```python
from build123d import *

# Parameters (mm, degrees)
EXTRUDE_1_DEPTH        = 2.9
SKETCH_2_R             = 2.75
EXTRUDE_2_DEPTH        = 5
FILLET_2_R             = 0.7
HOLE_WIZARD_M3_1_D     = 2.5
HOLE_WIZARD_M3_1_DEPTH = 10.1
HOLE_WIZARD_M3_1_TIP   = 0.751075774
FILLET_4_R             = 0.2


with BuildPart() as part:
    # 草图1 → 凸台-拉伸1 (new body)
    with BuildSketch(Plane(origin=(0, 0, 0), x_dir=(1, 0, 0), z_dir=(0, 1, 0))):
        Polygon((2.75, -1.58771324), (2.75, 1.58771324), (0, 3.175426481), (-2.75, 1.58771324), (-2.75, -1.58771324), (0, -3.175426481), align=None)
    extrude(amount=EXTRUDE_1_DEPTH)

    # 草图2 → 凸台-拉伸2 (add)
    with BuildSketch(Plane(origin=(0, 0, 0), x_dir=(-1, 0, 0), z_dir=(0, -1, 0))):
        with Locations(Location((0, 0, 0), (0, 0, 90))):
            Circle(SKETCH_2_R)
    extrude(amount=-EXTRUDE_2_DEPTH)

    # 圆角2
    fillet_2_edges = [part.edges().sort_by_distance(p)[0] for p in [
        (0, 5, 2.75),
    ]]
    fillet(fillet_2_edges, radius=FILLET_2_R)

    # M3 螺纹孔1
    with Locations(Plane(origin=(0, 0, 0), x_dir=(-1, 0, 0), z_dir=(0, -1, 0))):
        with Locations((0, 0)):
            Hole(HOLE_WIZARD_M3_1_D / 2, depth=HOLE_WIZARD_M3_1_DEPTH)
            with Locations((0, 0, -(HOLE_WIZARD_M3_1_DEPTH + HOLE_WIZARD_M3_1_TIP / 2))):  # 118° drill point
                Cone(0, HOLE_WIZARD_M3_1_D / 2, HOLE_WIZARD_M3_1_TIP, mode=Mode.SUBTRACT)

    # 圆角4
    fillet_4_edges = [part.edges().sort_by_distance(p)[0] for p in [
        (0, 1.45, 3.175426481),
        (-2.75, 1.45, 1.58771324),
        (-2.75, 1.45, -1.58771324),
        (0, 1.45, -3.175426481),
        (2.75, 1.45, -1.58771324),
        (2.75, 1.45, 1.58771324),
    ]]
    fillet(fillet_4_edges, radius=FILLET_4_R)


solid = part.part
```
Input: part model. Units: mm. Frame: model coordinates. A direction names the side the tool comes from. Give positions to 0.01 mm unless a question says otherwise; leave off trailing zeros. Order: outer loops, then holes, each group sorted by start corner. A loop starts at its lowest first (then second) coordinate and runs counter-clockwise, first axis right, second up. Notation, with made-up numbers: (9.25, 48) -> (38.25, 48) arc R19 ccw to (38.25, 55) -> close; hole circle Ø2 at (-21.75, 30.25). An arc over 180 degrees is marked (long way). Write each question's results on one line, items separated by ' | '. Start each with the question number.
Item 1: Contact query for flat-ended pins moving along their axis: P1, Ø0.6, axis at x = 0.5, z = 2.5, coming from the +Y side; P2, Ø1.5, axis at x = -1, y = 3.5, coming from the -Z side; P3, Ø0.7, axis at x = 2.5, z = -1.5, coming from the +Y side. Output: stop coordinate, or through.
Item 2: Cut plane A-A on x = 0. Return the cut outline in (y, z).
Item 3: Mould query, pull axis X, two halves, no side actions, for faces 6 (the flat face through (2.75, 1, 0)), 7 (the flat face through (-2.75, 1, 0)), 8 (the cylindrical face through (-0.27, 2.54, 1.22)). Classes: pulls with the +X half, pulls with the -X half, needs draft (parallel to the pull), parting line crosses it, or undercut.
Item 4: Cut plane B-B on y = 1.4. Return the cut outline in (x, z), then the cut area to 3 significant figures.
Item 5: Set-up query: faces 1 (the cylindrical face through (-2.685, 3.59, 0.596)), 2 (the flat face through (-2.52, 2.9, 1.45)), 3 (the flat face through (-2.5, 2.9, -1.5)), 4 (the flat face through (2.5, 2.9, -1.5)), 5 (the flat face through (2.52, 2.9, 1.45)). Return all of +Z, -Z, +X, -X, +Y, -Y with unobstructed straight access to the full face (end or side cutting, diameter ignored); none if empty.
Item 6: Cut plane C-C on y = 4.2. Return the cut outline in (x, z), then the cut area to 3 significant figures.
Item 7: Line query: line 1 (Z direction, x = 0, y = 1.05); line 2 (Z direction, x = -0.9, y = 3.15); line 3 (X direction, y = 4.35, z = -1). Output: solid intervals per line, ascending.
Established:
1) P1: y = 4.97 | P2: z = -2.86 | P3: y = 4.77
2) outline: (0, -3.14) -> (2.9, -3.14) -> (2.9, -2.75) -> (4.3, -2.75) arc R0.7 ccw to (5, -2.05) -> (5, -1.25) -> (0, -1.25) -> close; (0, 1.25) -> (5, 1.25) -> (5, 2.05) arc R0.7 ccw to (4.3, 2.75) -> (2.9, 2.75) -> (2.9, 3.14) -> (0, 3.14) -> close
3) face 6: pulls with the +X half | face 7: pulls with the -X half | face 8: undercut
4) outline: (-2.75, -1.47) arc R0.2 ccw to (-2.65, -1.65) -> (-0.1, -3.12) arc R0.2 ccw to (0.1, -3.12) -> (2.65, -1.65) arc R0.2 ccw to (2.75, -1.47) -> (2.75, 1.47) arc R0.2 ccw to (2.65, 1.65) -> (0.1, 3.12) arc R0.2 ccw to (-0.1, 3.12) -> (-2.65, 1.65) arc R0.2 ccw to (-2.75, 1.47) -> close; hole circle Ø2.5 at (0, 0) | area: 21.3 mm^2
5) face 1: +Y | face 2: +Z, -X, +Y | face 3: -Z, -X, +Y | face 4: -Z, +X, +Y | face 5: +Z, +X, +Y
6) outline: circle Ø5.5 at (0, 0); hole circle Ø2.5 at (0, 0) | area: 18.8 mm^2
7) line 1: -3.14 to -1.25, 1.25 to 3.14 | line 2: -2.6 to -0.87, 0.87 to 2.6 | line 3: -2.56 to -0.75, 0.75 to 2.56
